```python
from build123d import *

# Parameters (mm, degrees)
SKETCH1_W           = 152.4
SKETCH1_H           = 152.4
BOSS_EXTRUDE1_DEPTH = 50
SKETCH2_R           = 6
CUT_EXTRUDE1_DEPTH  = 178.573083546
SKETCH4_R           = 6
CUT_EXTRUDE2_DEPTH  = 178.573083546


with BuildPart() as part:
    # Sketch1 → Boss-Extrude1 (new body)
    with BuildSketch(Plane.XY):
        Rectangle(SKETCH1_W, SKETCH1_H)
    extrude(amount=BOSS_EXTRUDE1_DEPTH)

    # Sketch2 → Cut-Extrude1 (cut, through all)
    with BuildSketch(Plane(origin=(76.2, 0, 0), x_dir=(0, 0, -1), z_dir=(1, 0, 0))):
        with Locations(Location((-40, 56.2, 0), (0, 0, 90))):
            Circle(SKETCH2_R)
        with Locations(Location((-40, 0, 0), (0, 0, 90))):
            Circle(SKETCH2_R)
        with Locations(Location((-40, -56.2, 0), (0, 0, 90))):
            Circle(SKETCH2_R)
    extrude(amount=-CUT_EXTRUDE1_DEPTH, mode=Mode.SUBTRACT)

    # Sketch4 → Cut-Extrude2 (cut, through all)
    with BuildSketch(Plane(origin=(0, 76.2, 0), x_dir=(1, 0, 0), z_dir=(0, 1, 0))):
        with Locations(Location((-56.2, -10, 0), (0, 0, 270))):
            Circle(SKETCH4_R)
        with Locations(Location((0, -10, 0), (0, 0, 270))):
            Circle(SKETCH4_R)
        with Locations(Location((56.2, -10, 0), (0, 0, 270))):
            Circle(SKETCH4_R)
    extrude(amount=-CUT_EXTRUDE2_DEPTH, mode=Mode.SUBTRACT)


solid = part.part
```
Can you work these out from the model? Positions are in its coordinate system, mm. Coordinates: 2 decimals unless noted, no trailing zeros. Loops run counter-clockwise (first coordinate to the right, second up) from the corner with the lowest first, then second, coordinate; pieces in that order, holes last.
Item 1: Please list where these lines run through material, in increasing order: L1, parallel to Y at x = -48, z = 43; L2, parallel to Z at x = 56.5, y = -35; L3, parallel to Z at x = 5.5, y = -56.2.
Answers below:
L1: y = -76.2 to -61.4, -51 to -5.2, 5.2 to 51, 61.4 to 76.2
L2: z = 0 to 4.01, 15.99 to 50
L3: z = 0 to 7.6, 12.4 to 34, 46 to 50
Item 2: Suppose I cut it at A-A (y = 0). Please give me the cut outline in (x, z), then the cut area to 3 significant figures.
Answers below:
outline: (-76.2, 0) - (76.2, 0) - (76.2, 34) - (-76.2, 34) - close; (-76.2, 46) - (76.2, 46) - (76.2, 50) - (-76.2, 50) - close; hole circle Ø12 at (-56.2, 10); hole circle Ø12 at (0, 10); hole circle Ø12 at (56.2, 10)
area: 5,450 mm2
Item 3: Suppose I cut it at D-D (x = 0). Please give me the cut outline in (y, z), then the cut area to 3 significant figures.
Answers below:
outline: (-76.2, 0) - (76.2, 0) - (76.2, 4) - (-76.2, 4) - close; (-76.2, 16) - (76.2, 16) - (76.2, 50) - (-76.2, 50) - close; hole circle Ø12 at (-56.2, 40); hole circle Ø12 at (0, 40); hole circle Ø12 at (56.2, 40)
area: 5,450 mm2
Item 4: If we mould it in two halves opening along X, with no side actions, what happens to faces 1 (the face through (76.2, -1, 25)), 2 (the face through (-1, -76.2, 25)), 3 (the face through (-62.057, 1.067, 8.699))? For each: released by +X, released by -X, zero draft, split by the parting line, or undercut.
Answers below:
face 1: released by +X
face 2: zero draft
face 3: undercut
Item 5: Suppose I cut it at B-B (z = 10). Please give me the cut outline in (x, y), then the cut area to 3 significant figures.
Answers below:
outline: (-76.2, -76.2) - (-62.2, -76.2) - (-62.2, 76.2) - (-76.2, 76.2) - close; (-50.2, -76.2) - (-6, -76.2) - (-6, 76.2) - (-50.2, 76.2) - close; (6, -76.2) - (50.2, -76.2) - (50.2, 76.2) - (6, 76.2) - close; (62.2, -76.2) - (76.2, -76.2) - (76.2, 76.2) - (62.2, 76.2) - close
area: 17,700 mm2
Item 6: Suppose I cut it at C-C (x = -31.5). Please give me the cut outline in (y, z), then the cut area to 3 significant figures.
Answers below:
outline: (-76.2, 0) - (76.2, 0) - (76.2, 50) - (-76.2, 50) - close; hole circle Ø12 at (-56.2, 40); hole circle Ø12 at (0, 40); hole circle Ø12 at (56.2, 40)
area: 7,280 mm2
